The listing builds one solid part. Answer for the finished solid, in the listing's coordinates (mm). A direction names the side the tool comes from. Give positions to 0.01 mm unless a question says otherwise; leave off trailing zeros. Order: outer loops, then holes, each group sorted by start corner. A loop starts at its lowest first (then second) coordinate and runs counter-clockwise, first axis right, second up. Notation, with made-up numbers: (14.5, 49.25) -> (42.5, 49.25) arc R29 ccw to (42.5, 72.25) -> close; hole circle Ø9 at (50.25, 23). An arc over 180 degrees is marked (long way). Answer as a JSON object with one key per item and string values. Group by question number.
Solid Edge part; units mm, degrees
sketch "Sketch1" plane through (0, 0, 0) normal (0, 0, 1) x (1, 0, 0)
  circle A0 centre (0, 0) radius 4
extrude "Protrusion1" add sketch "Sketch1" along normal mid plane 8
chamfer "Chamfer1" distance 0.6 angle 45 2 edges at (-4, 0, -4) (-4, 0, 4)
sketch "Sketch2" plane through (0, 0, 4) normal (0, 0, 1) x (1, 0, 0)
  line L0 (-1.1547, 2) -> (1.1547, 2)
  line L1 (2.3094, 0) -> (1.1547, 2)
  line L2 (1.1547, -2) -> (2.3094, 0)
  line L3 (-1.1547, -2) -> (1.1547, -2)
  line L4 (-2.3094, 0) -> (-1.1547, -2)
  line L5 (-1.1547, 2) -> (-2.3094, 0)
extrude "Cutout1" cut sketch "Sketch2" against normal blind 4
properties part number "24104459"
(1) Which of the six approach directions +Z, -Z, +X, -X, +Y, -Y give full straight-line access (tool end or side, diameter ignored) to faces 1 (the flat face through (-2, -1, 4)), 2 (the flat face through (0, 0, 0))?
(2) A cutting plane is placed at C-C (z = -2.5). Determine the outline of the cut face in (x, y), and give its area (3 significant figures).
(3) Find the intervals of material crossed by line 1 along Y through (x, z) = (0, 1.5); line 2 along Z through (x, y) = (-0.5, 0.5); line 3 along X through (y, z) = (-1.5, 1.75), in increasing order. Write a range as [from, to].
(4) A cutting plane is placed at A-A (z = 1.75). Determine the outline of the cut face in (x, y), and give its area (3 significant figures).
(5) For a pull along X with two mould halves and no side action, classify faces 3 (the cylindrical face through (-0.867, 3.905, -0.048)), 4 (the flat face through (0, 0, -4)), 5 (the flat face through (0, -2, 2)), 6 (the flat face through (1.724, -1.014, 2.028)) as +X half, -X half, draft (parallel to the pull), parting line (faces both ways), or undercut.
(6) Flat-ended cylindrical pins translate along their axes: pin 1 Ø0.7 at (x, z) = (-0.5, 1) entering from +Y; pin 2 Ø1.2 at (x, y) = (0.5, -0.5) entering from +Z. Find the tip coordinate at first contact, or state that the pin passes through.
(7) A cutting plane is placed at B-B (x = 0). Determine the outline of the cut face in (y, z), and give its area (3 significant figures).
Check sheet entries:
{
 "1": {"face 1": "+Z, +X, -X, +Y, -Y", "face 2": "+Z"},
 "2": {"outline": "circle Ø8 at (0, 0)", "area": "50.3 mm2"},
 "3": {"line 1": "y = [-4, -2], [2, 4]", "line 2": "z = [-4, 0]", "line 3": "x = [-3.71, -1.44], [1.44, 3.71]"},
 "4": {"outline": "circle Ø8 at (0, 0); hole (-2.31, 0) -> (-1.15, -2) -> (1.15, -2) -> (2.31, 0) -> (1.15, 2) -> (-1.15, 2) -> close", "area": "36.4 mm2"},
 "5": {"face 3": "parting line", "face 4": "draft", "face 5": "undercut", "face 6": "undercut"},
 "6": {"pin 1": "stops at y = 4", "pin 2": "stops at z = 0"},
 "7": {"outline": "(-4, -3.4) -> (-3.4, -4) -> (3.4, -4) -> (4, -3.4) -> (4, 3.4) -> (3.4, 4) -> (2, 4) -> (2, 0) -> (-2, 0) -> (-2, 4) -> (-3.4, 4) -> (-4, 3.4) -> close", "area": "47.3 mm2"}
}
